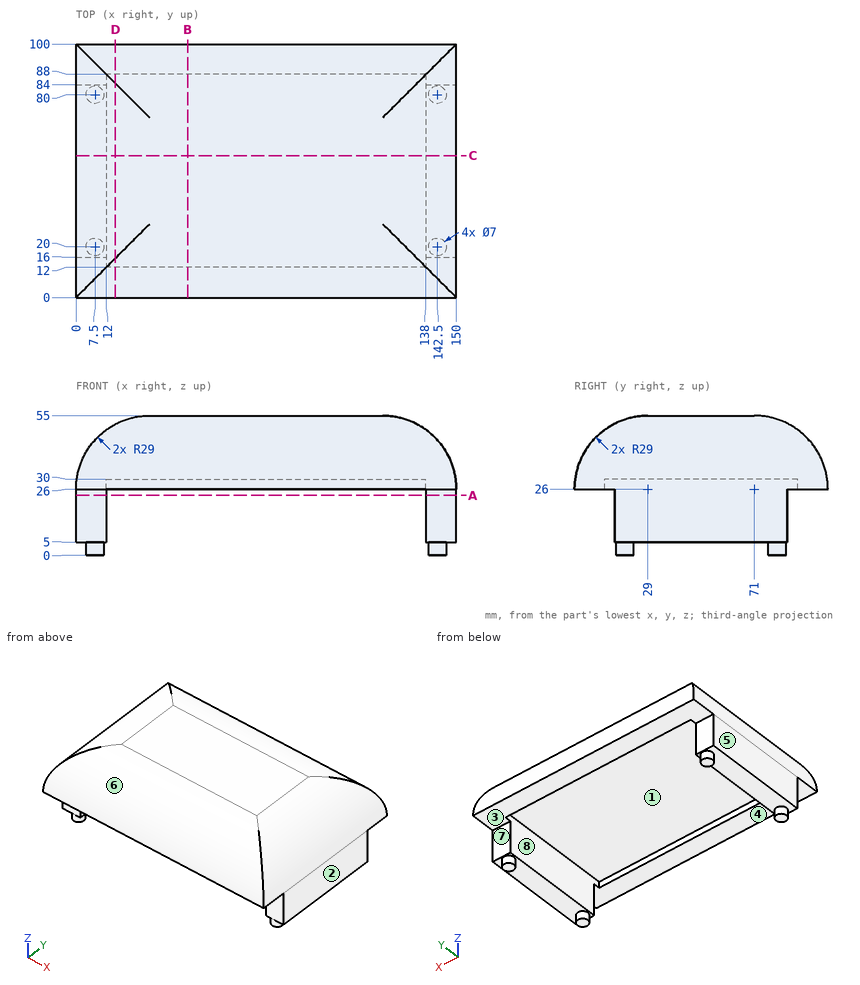
Job drawing, mm, ordinate dimensions from the low corner. One solid piece. A direction names the side the tool comes from. Coordinates: 2 decimals unless noted, no trailing zeros. Order: outer loops, then holes, each group sorted by start corner. A loop starts at its lowest first (then second) coordinate and runs counter-clockwise, first axis right, second up. Notation, with made-up numbers: (61.5, 28) -> (109.5, 28) arc R24 cw to (109.5, 60) -> close; hole circle Ø3 at (8.25, -23). An arc over 180 degrees is marked (long way). Answer in a Markdown table with one row per item. Add a question column.
Q1. Band-saw the part on B-B, the plane x = 44. List the corners of the cut face in (y, z).
Q2. Band-saw the part on A-A, the plane z = 23.5. List the corners of the cut face in (x, y), then the cut area to 3 significant figures.
Q3. Band-saw the part on D-D, the plane x = 15.5. List the corners of the cut face in (y, z).
Q4. Mould opens along X. For the marked faces 1, 2 and 3 say: +X half, -X half, draft (parallel to the pull), parting line (faces both ways), or undercut.
Q5. Which spindle directions (+Z, -Z, +X, -X, +Y, -Y) get a long thin tool onto all of the face, cutting with end or side? Do the marked faces 4, 5, 6, 7 and 8. Say none if no direction does.
Q6. Wall check: line 1 along X through (y, z) = (50, 20); line 2 along Z through (x, y) = (29, 46.5); line 3 along Z through (x, y) = (104.5, 14). Give the ranges that are in metal, low to high. Write a range as [from, to].
Q7. Band-saw the part on C-C, the plane y = 56. List the corners of the cut face in (x, z), then the cut area to 3 significant figures.
Q8. Drop flat-ended pins along their axis: pin 1 (23 mm diameter, centred on x = 59, y = 42, fed in from -Z); pin 2 (3.5 mm diameter, centred on x = 145, z = 16.5, fed in from -Y); pin 3 (8 mm diameter, centred on x = 91, z = 30.5, fed in from -Y). Give the stop position or say it passes through.
Answers follow:
| question | item | result |
|---|---|---|
| 1 | outline | (0, 26) -> (12, 26) -> (12, 30) -> (88, 30) -> (88, 26) -> (100, 26) arc R29 ccw to (71, 55) -> (29, 55) arc R29 ccw to start |
| 2 | outline | (0, 16) -> (12, 16) -> (12, 84) -> (0, 84) -> close; (138, 16) -> (150, 16) -> (150, 84) -> (138, 84) -> close |
| 2 | area | 1,630 mm^2 |
| 3 | outline | (0, 26) -> (12, 26) -> (12, 30) -> (88, 30) -> (88, 26) -> (100, 26) arc R29 ccw to (84.5, 51.67) -> (15.5, 51.67) arc R29 ccw to start |
| 4 | face 1 | undercut |
| 4 | face 2 | +X half |
| 4 | face 3 | draft |
| 5 | face 4 | -Z, +X, -X, -Y |
| 5 | face 5 | +Z, -Z, -X, +Y, -Y |
| 5 | face 6 | +Z, +X, -X, -Y |
| 5 | face 7 | -Z, +X, -X, +Y |
| 5 | face 8 | -Z |
| 6 | line 1 | [0, 12], [138, 150] |
| 6 | line 2 | [30, 55] |
| 6 | line 3 | [30, 50.82] |
| 7 | outline | (0, 5) -> (12, 5) -> (12, 30) -> (138, 30) -> (138, 5) -> (150, 5) -> (150, 26) arc R29 ccw to (121, 55) -> (29, 55) arc R29 ccw to (0, 26) -> close |
| 7 | area | 3,990 mm^2 |
| 8 | pin 1 | z = 30 |
| 8 | pin 2 | y = 16 |
| 8 | pin 3 | y = 0 |
